from build123d import *

# Parameters (mm, degrees)
F0_W     = 50.8
F0_H     = 76.2
F1_DEPTH = 12.7
F2_R     = 17.78
F3_DEPTH = 25.4
F4_R     = 17.78
F5_DEPTH = 25.4
F6_W     = 2.54
F6_H     = 10.16
F7_DEPTH = 25.4
F8_W     = 2.54
F8_H     = 10.16
F9_DEPTH = 25.4


with BuildPart() as f1:
    # F0 (on Top) → F1 (new body)
    with BuildSketch(Plane.XY):
        Rectangle(F0_W, F0_H)
    extrude(amount=F1_DEPTH)

    # F2 (on face) → F3 (cut)
    with BuildSketch(Plane.XY.offset(12.7)):
        with Locations((25.4, 0)):
            Circle(F2_R)
    extrude(amount=-F3_DEPTH, mode=Mode.SUBTRACT)

    # F4 (on face) → F5 (cut)
    with BuildSketch(Plane.XY.offset(12.7)):
        with Locations((-25.4, 0)):
            Circle(F4_R)
    extrude(amount=-F5_DEPTH, mode=Mode.SUBTRACT)

    # F6 (on face) → F7 (cut)
    with BuildSketch(Plane.XY.offset(12.7)):
        with Locations((4.96473, 33.02)):
            Rectangle(F6_W, F6_H)
    extrude(amount=-F7_DEPTH, mode=Mode.SUBTRACT)

    # F8 (on face) → F9 (cut)
    with BuildSketch(Plane.XY.offset(12.7)):
        with Locations((-4.718008, 33.746003)):
            Rectangle(F8_W, F8_H)
    extrude(amount=-F9_DEPTH, mode=Mode.SUBTRACT)


solid = f1.part
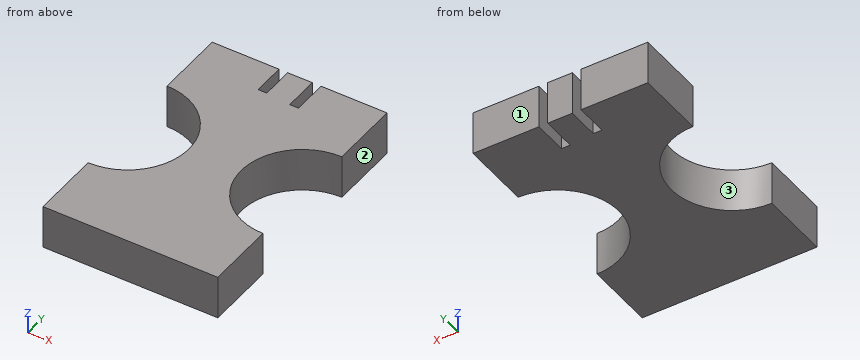
For this review, take the finished solid that the model builds, in its own axes (mm). Face numbers are marked on the shaded views. Coordinates: 2 decimals unless noted, no trailing zeros. Loops run counter-clockwise (first coordinate to the right, second up) from the corner with the lowest first, then second, coordinate; pieces in that order, holes last. Notation, with made-up numbers: (28, 37) -> (76, 37) arc R22 ccw to (76, 76) -> close; hole circle Ø7 at (-4, -24). An arc over 180 degrees is marked (long way). Write each question's results on one line, items separated by ' | '.
Q1. Mouldability with a two-part tool opening along Y and no side actions: class the marked faces 1, 2 and 3 as +Y half, -Y half, draft (parallel to the pull), parting line (faces both ways), or undercut.
Taken from the geometry:
face 1: +Y half | face 2: draft | face 3: undercut
Q2. Add section D-D, the plane x = -4.5. State the section outline as (y, z) points.
Taken from the geometry:
outline: (-38.1, 0) -> (28.67, 0) -> (28.67, 12.7) -> (-38.1, 12.7) -> close
Q3. Add section B-B, the plane z = 4.5. State the section outline as (x, y) points, then the cut area to 3 significant figures.
Taken from the geometry:
outline: (-25.4, -38.1) -> (25.4, -38.1) -> (25.4, -17.78) arc R17.78 cw to (25.4, 17.78) -> (25.4, 38.1) -> (6.23, 38.1) -> (6.23, 27.94) -> (3.69, 27.94) -> (3.69, 38.1) -> (-3.45, 38.1) -> (-3.45, 28.67) -> (-5.99, 28.67) -> (-5.99, 38.1) -> (-25.4, 38.1) -> (-25.4, 17.78) arc R17.78 cw to (-25.4, -17.78) -> close | area: 2,830 mm²
Q4. To check wall thickness, follow line 1 along X through (y, z) = (34.5, 7.25); line 2 along Y through (x, z) = (4.5, 7.25); line 3 along Y through (x, z) = (11, 2.5). State the ranges of each line that lie inside material, in increasing order. Write a range as [from, to].
Taken from the geometry:
line 1: [-25.4, -5.99], [-3.45, 3.69], [6.23, 25.4] | line 2: [-38.1, 27.94] | line 3: [-38.1, -10.43], [10.43, 38.1]
Q5. For pin 1 Ø1 at (y, z) = (-3.5, 3) entering from +X; pin 2 Ø2 at (x, z) = (-4.5, 7) entering from +Y; pin 3 Ø2 at (y, z) = (-12.5, 7) entering from +X, all flat-tipped, find the tip position at first contact; note any pin that passes through.
Taken from the geometry:
pin 1: x = 8.08 | pin 2: y = 28.67 | pin 3: x = 13.83
Q6. Add section A-A, the plane x = 8.5. State the section outline as (y, z) points, then the cut area to 3 significant figures.
Taken from the geometry:
outline: (-38.1, 0) -> (-5.52, 0) -> (-5.52, 12.7) -> (-38.1, 12.7) -> close; (5.52, 0) -> (38.1, 0) -> (38.1, 12.7) -> (5.52, 12.7) -> close | area: 827 mm²
Q7. Add section C-C, the plane y = 0. State the section outline as (x, z) points, then the cut area to 3 significant figures.
Taken from the geometry:
outline: (-7.62, 0) -> (7.62, 0) -> (7.62, 12.7) -> (-7.62, 12.7) -> close | area: 194 mm²
